```python
from build123d import *

# Parameters (mm, degrees)
BOSS_EXTRUDE1_DEPTH = 2
SKETCH2_R           = 1.5
SKETCH2_R_2         = 5.625
CUT_EXTRUDE1_DEPTH  = 2
CUT_EXTRUDE2_DEPTH  = 2


with BuildPart() as part:
    # Sketch1 → Boss-Extrude1 (new body)
    with BuildSketch(Plane(origin=(0, 0, 0), x_dir=(1, 0, 0), z_dir=(0, 1, 0))):
        Polygon((2.75, 52), (-2.75, 52), (-4.5, 50.25), (-9.984901653, 50.25), (-11.5, 54), (-21, 48.515172443), (-21, 38.719848481), (-18.65, 36.369848481), (-18.65, 20.319848481), (-21, 17.969848481), (-21, 6.969848481), (-18.030151519, 4), (-15.17820323, 4), (-8.25, 0), (8.25, 0), (15.17820323, 4), (18.030151519, 4), (21, 6.969848481), (21, 17.969848481), (18.65, 20.319848481), (18.65, 36.369848481), (21, 38.719848481), (21, 48.515172443), (11.5, 54), (9.984901653, 50.25), (4.5, 50.25), align=None)
    extrude(amount=BOSS_EXTRUDE1_DEPTH)

    # Sketch2 → Cut-Extrude1 (cut)
    with BuildSketch(Plane(origin=(0, 2, 0), x_dir=(1, 0, 0), z_dir=(0, 1, 0))):
        with Locations(Location((-17.713628621, 45.005868893, 0), (0, 0, 270))):
            Circle(SKETCH2_R)
        with Locations(Location((-17.443074505, 7.627226222, 0), (0, 0, 270))):
            Circle(SKETCH2_R)
        with Locations(Location((0, 10.45, 0), (0, 0, 270))):
            Circle(SKETCH2_R)
        with Locations(Location((0, 17, 0), (0, 0, 270))):
            Circle(SKETCH2_R)
        with Locations(Location((0, 26.375, 0), (0, 0, 270))):
            Circle(SKETCH2_R_2)
        with Locations(Location((-8.82739896, 17.75936, 0), (0, 0, 270))):
            Circle(SKETCH2_R)
        with Locations(Location((-7.925, 26.375, 0), (0, 0, 270))):
            Circle(SKETCH2_R)
        with Locations(Location((-13.890686283, 34.212926204, 0), (0, 0, 270))):
            Circle(SKETCH2_R)
        with Locations(Location((-8.829730603, 34.988250401, 0), (0, 0, 270))):
            Circle(SKETCH2_R)
        with Locations(Location((0, 35.72, 0), (0, 0, 270))):
            Circle(SKETCH2_R)
    cut_extrude1 = extrude(amount=-CUT_EXTRUDE1_DEPTH, mode=Mode.SUBTRACT)

    # Mirror1: Cut-Extrude1 across plane
    add(cut_extrude1.mirror(Plane(origin=(0, 0, 0), x_dir=(0, 0, 1), z_dir=(1, 0, 0))), mode=Mode.SUBTRACT)

    # Sketch3 → Cut-Extrude2 (cut)
    with BuildSketch(Plane(origin=(0, 2, 0), x_dir=(1, 0, 0), z_dir=(0, 1, 0))):
        with BuildLine():
            Line((-2.486814901, 47.397027552), (-12.935032384, 48.224828091))
            ThreePointArc((-12.935032384, 48.224828091), (-13.64734637, 47.894907892), (-13.734631847, 47.114767008))
            Line((-13.734631847, 47.114767008), (-10.820083793, 40.247881869))
            ThreePointArc((-10.820083793, 40.247881869), (-10.542892619, 39.905374095), (-10.126394281, 39.761583775))
            Line((-10.126394281, 39.761583775), (-2.592724852, 39.358665124))
            ThreePointArc((-2.592724852, 39.358665124), (-1.999627345, 39.576928954), (-1.75, 40.157523426))
            Line((-1.75, 40.157523426), (-1.75, 46.599526679))
            ThreePointArc((-1.75, 46.599526679), (-1.962399762, 47.142413371), (-2.486814901, 47.397027552))
        make_face()
        with BuildLine():
            Line((10.126394281, 39.761583775), (2.592724852, 39.358665124))
            ThreePointArc((2.592724852, 39.358665124), (1.999627345, 39.576928954), (1.75, 40.157523426))
            Line((1.75, 40.157523426), (1.75, 46.599526679))
            ThreePointArc((1.75, 46.599526679), (1.962399762, 47.142413371), (2.486814901, 47.397027552))
            Line((2.486814901, 47.397027552), (12.935032384, 48.224828091))
            ThreePointArc((12.935032384, 48.224828091), (13.64734637, 47.894907892), (13.734631847, 47.114767008))
            Line((13.734631847, 47.114767008), (10.820083793, 40.247881869))
            ThreePointArc((10.820083793, 40.247881869), (10.542892619, 39.905374095), (10.126394281, 39.761583775))
        make_face()
    extrude(amount=-CUT_EXTRUDE2_DEPTH, mode=Mode.SUBTRACT)


solid = part.part
```
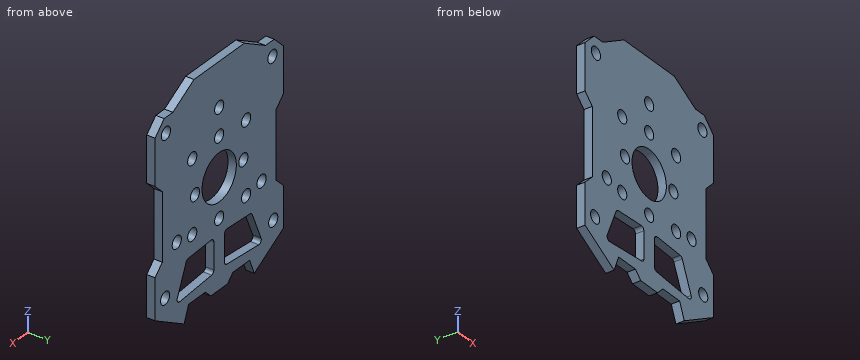
The listing builds one solid part. Answer for the finished solid, in the listing's coordinates (mm). Coordinates: 2 decimals unless noted, no trailing zeros. Loops run counter-clockwise (first coordinate to the right, second up) from the corner with the lowest first, then second, coordinate; pieces in that order, holes last. Notation, with made-up numbers: (85, -0.5) - (94, -0.5) arc R19 cw to (94, 14.5) - close; hole circle Ø5 at (-1, -15.75). An arc over 180 degrees is marked (long way). Write item = value, one per line.
1) Section B-B (z = -10.45) is taken. Determine the outline of the cut face in (x, y).
Responses:
outline = (-21, 0) - (-1.5, 0) - (-1.5, 2) - (-21, 2) - close; (1.5, 0) - (21, 0) - (21, 2) - (1.5, 2) - close
2) Section D-D (z = -28.5) is taken. Determine the outline of the cut face in (x, y).
Responses:
outline = (-18.65, 0) - (-5.21, 0) - (-5.21, 2) - (-18.65, 2) - close; (5.21, 0) - (18.65, 0) - (18.65, 2) - (5.21, 2) - close
3) Section C-C (z = -17) is taken. Determine the outline of the cut face in (x, y), plus the area to 3 significant figures.
Responses:
outline = (-21, 0) - (-10.12, 0) - (-10.12, 2) - (-21, 2) - close; (-7.53, 0) - (-1.5, 0) - (-1.5, 2) - (-7.53, 2) - close; (1.5, 0) - (7.53, 0) - (7.53, 2) - (1.5, 2) - close; (10.12, 0) - (21, 0) - (21, 2) - (10.12, 2) - close
area = 67.7 mm^2
4) Each of these flat-tipped pins is pushed along its axis until it touches: P1, Ø0.6, axis at x = 7, y = 1, coming from the -Z side; P2, Ø0.6, axis at y = 1, z = -27, coming from the +X side. Where does it stop, or does it pass through?
Responses:
P1 = -50.25
P2 = 18.65
5) Section A-A (x = 0) is taken. Determine the outline of the cut face in (y, z), plus the area to 3 significant figures.
Responses:
outline = (0, -52) - (2, -52) - (2, -37.22) - (0, -37.22) - close; (0, -34.22) - (2, -34.22) - (2, -32) - (0, -32) - close; (0, -20.75) - (2, -20.75) - (2, -18.5) - (0, -18.5) - close; (0, -15.5) - (2, -15.5) - (2, -11.95) - (0, -11.95) - close; (0, -8.95) - (2, -8.95) - (2, 0) - (0, 0) - close
area = 63.5 mm^2
6) Find the intervals of material crossed by line 1 along X through (y, z) = (1.05, -7.5); line 2 along Z through (x, y) = (-9, 0.3); line 3 along X through (y, z) = (0.5, -43), in increasing order.
Responses:
line_1 = -21 to -18.94, -15.95 to 15.95, 18.94 to 21
line_2 = -50.25 to -47.91, -39.7 to -36.48, -33.5 to -27.42, -25.33 to -19.25, -16.27 to -0.43
line_3 = -21 to -11.99, -1.75 to 1.75, 11.99 to 21
